For this review, take the finished solid that the model builds, in its own axes (mm). A direction names the side the tool comes from. Round coordinates to 2 decimals unless told otherwise and drop trailing zeros. Order: outer loops, then holes, each group sorted by start corner. A loop starts at its lowest first (then second) coordinate and runs counter-clockwise, first axis right, second up. Notation, with made-up numbers: (68.5, 43) -> (84.5, 43) arc R16 cw to (84.5, 70) -> close; hole circle Ø10 at (69.5, 51). An arc over 180 degrees is marked (long way). Answer in a Markdown table with one row per item.
Autodesk Inventor part; units mm, degrees
sketch "Skizze1" plane through (0, 0, 0) normal (0, 0, 1) x (1, 0, 0)
  circle A0 centre (0, 0) radius 21
  line L0 (-16.8526, 12.5296) -> (0, 0)
  line L1 (0, 0) -> (-8.33, 19.2772)
  line L2 (0, 0) -> (8.0192, 19.4086)
  line L3 (0, 0) -> (18.1865, 10.5)
  line L4 (0, 0) -> (21, 0) construction
  line L5 (0, 0) -> (-13.5496, -16.044)
  line L6 (0, 0) -> (13.0769, -16.4315)
  circle A1 centre (0, 0) radius 27.5
  circle A2 centre (0, 0) radius 12.5
  line L7 (-27.5, 11.3909) -> (-11.3909, 27.5)
  line L8 (-11.3909, 27.5) -> (11.3909, 27.5)
  line L9 (11.3909, 27.5) -> (27.5, 11.3909)
  line L10 (27.5, 11.3909) -> (27.5, -11.3909)
  line L11 (27.5, -11.3909) -> (11.3909, -27.5)
  line L12 (11.3909, -27.5) -> (-11.3909, -27.5)
  line L13 (-11.3909, -27.5) -> (-27.5, -11.3909)
  line L14 (-27.5, -11.3909) -> (-27.5, 11.3909)
  circle A3 centre (0, 0) radius 3.25
  point P0 (0, 0)
  point P1 (-27.5, 0)
  dimension "d3" = 55
  dimension "d0" = 42
  dimension "d1" = 30
  dimension "d2" = 30
  dimension "d4" = 25
  dimension "d27" = 0
  dimension "d28" = 0
  dimension "d105" = 6.5
extrude "Extrusion21" add sketch "Skizze1" along normal blind 53 contours A0 L6 A2 L3 | L3 A2 L2 A0 | A0 L5 A2 L6 | L2 A2 L1 A0 | A2 L6 A3 L3 | L3 A3 L2 A2 | A0 L0 A2 L5 | A2 L5 A3 L6 | L1 A2 L0 A0 | L2 A3 L1 A2 | A3 L6 L3 | L3 L2 A3 | A2 L0 A3 L5 | A3 L5 L6 | L1 A3 L0 A2 | L2 L1 A3 | L5 A3 L0 | L0 A3 L1 | A1 | L10 L11 A1 | A1 L9 L10 | A1 L8 L9 | L11 L12 A1 | A1 L7 L8 | L12 L13 A1 | A1 L14 L7 | L13 L14 A1
sketch "Skizze18" plane through (0, 0, 0) normal (0, 0, 1) x (1, 0, 0)
  line L0 (-11.3909, 27.5) -> (11.3909, 27.5)
  line L1 (-11.3909, 27.5) -> (63.1653, 27.5)
  line L2 (63.1653, 27.5) -> (63.1653, -27.5)
  line L3 (63.1653, -27.5) -> (-11.3909, -27.5)
  line L4 (-11.3909, -27.5) -> (-11.3909, 27.5)
  point P0 (0, 0)
  dimension "d154" = 55
extrude "Extrusion22" cut sketch "Skizze18" along normal through all
sketch "Skizze19" plane through (0, 0, 0) normal (1, 0, 0) x (0, 1, 0)
  line L0 (12.25, 9.875) -> (-12.25, 9.875)
  line L1 (-12.25, 9.875) -> (-12.25, 5.125)
  line L2 (-12.25, 5.125) -> (12.25, 5.125)
  line L3 (12.25, 5.125) -> (12.25, 9.875)
  line L4 (27.5, 0) -> (-27.5, 0)
  line L5 (-27.5, 0) -> (-27.5, 53)
  point P0 (0, 0)
  dimension "d157" = 24.5
  dimension "d158" = 4.75
  dimension "d159" = 5.125
  dimension "d160" = 39.75
sketch "Skizze20" plane through (0, 0, 0) normal (1, 0, 0) x (0, 1, 0)
  line L0 (-15, 48.125) -> (15, 48.125)
  line L1 (15, 48.125) -> (15, 42.875)
  line L2 (15, 42.875) -> (-15, 42.875)
  line L3 (-15, 42.875) -> (-15, 48.125)
  line L4 (5, 48.125) -> (-5, 48.125)
  line L5 (-5, 48.125) -> (-5, 42.875)
  line L6 (-5, 42.875) -> (5, 42.875)
  line L7 (5, 42.875) -> (5, 48.125)
  line L8 (-27.5, 53) -> (27.5, 53)
  point P0 (0, 0)
  dimension "d165" = 30
  dimension "d166" = 5.25
  dimension "d168" = 10
  dimension "d169" = 5.25
  dimension "d170" = 10
  dimension "d171" = 5
  dimension "d172" = 4.875
extrude "Extrusion23" cut sketch "Skizze20" against normal blind 20.5 contours L0 L5 L2 L3 | L0 L1 L2 L7
extrude "Extrusion25" add sketch "Skizze19" along normal blind 10 and the other way blind 25
fillet "Rundung11" radius 2 5 edges at (-19.4454, 19.4454, 53) (-27.5, 0, 53) (-19.4454, -19.4454, 53) (-27.5, -11.3909, 26.5) (-27.5, 11.3909, 26.5)
fillet "Rundung12" radius 1 12 edges at (-11.3909, 15, 45.5) (-11.3909, 10, 42.875) (-11.3909, 5, 45.5) (-11.3909, 10, 48.125) (-11.3909, -5, 45.5) (-11.3909, -10, 42.875) (-11.3909, -15, 45.5) (-11.3909, -10, 48.125) (10, 0, 9.875) (10, -12.25, 7.5) (10, 0, 5.125) (10, 12.25, 7.5)
sketch "Skizze22" plane through (0, 0, 0) normal (0, 1, 0) x (-1, 0, 0)
  line L0 (26.9142, 0) -> (11.3909, 0)
  line L1 (11.3909, 0) -> (11.3909, 51)
  line L2 (11.3909, 53) -> (25.5, 53)
  line L3 (-11.1091, 37.75) -> (-11.1091, 15.25)
  line L4 (11.3909, 15.25) -> (11.3909, 37.75)
  line L5 (11.3909, 37.75) -> (2.2757, 37.75)
  line L6 (-2.494, 37.75) -> (-11.1091, 37.75)
  arc A0 (-2.494, 37.75) -> (-2.494, 15.25) centre (-0.1091, 26.5) ccw
  arc A1 (2.2757, 15.25) -> (2.2757, 37.75) centre (-0.1091, 26.5) ccw
  line L7 (-11.1091, 15.25) -> (-2.494, 15.25)
  line L8 (2.2757, 15.25) -> (11.3909, 15.25)
  line L9 (11.3909, 0) -> (11.3909, 51)
  point P0 (0, 0)
  point P1 (11.3909, 26.5)
  dimension "d195" = 26.5
  dimension "d196" = 11.5
  dimension "d197" = 22.5
  dimension "d198" = 22.5
  dimension "d199" = 15.25
  dimension "d200" = 0
extrude "Extrusion26" cut sketch "Skizze1" along normal blind 20 contours A3 L6 L3 | L3 L2 A3 | A3 L5 L6 | L2 L1 A3 | L5 A3 L0 | L0 A3 L1
extrude "Extrusion28" add sketch "Skizze22" along normal mid plane 55 contours L8 A1 L1 | A1 L5 L1
sketch "Skizze12" plane through (0, 0, 14.5) normal (0, 0, 1) x (1, 0, 0)
  circle A0 centre (0, 0) radius 21
  line L0 (-16.8526, 12.5296) -> (-10.0313, 7.4581)
  line L1 (-4.9583, 11.4745) -> (-8.33, 19.2772)
  line L2 (4.7734, 11.5527) -> (8.0192, 19.4086)
  line L3 (10.8253, 6.25) -> (18.1865, 10.5)
  line L4 (0, 0) -> (21, 0) construction
  line L5 (-8.0652, -9.55) -> (-13.5496, -16.044)
  line L6 (7.7839, -9.7807) -> (13.0769, -16.4315)
  circle A1 centre (0, 0) radius 27.5
  circle A2 centre (0, 0) radius 12.5
  line L7 (-27.5, 11.3909) -> (-11.3909, 27.5)
  line L8 (-11.3909, 27.5) -> (11.3909, 27.5)
  line L9 (11.3909, 27.5) -> (27.5, 11.3909)
  line L10 (27.5, 11.3909) -> (27.5, -11.3909)
  line L11 (27.5, -11.3909) -> (11.3909, -27.5)
  line L12 (11.3909, -27.5) -> (-11.3909, -27.5)
  line L13 (-11.3909, -27.5) -> (-27.5, -11.3909)
  line L14 (-27.5, -11.3909) -> (-27.5, 11.3909)
  point P0 (0, 0)
  point P1 (-27.5, 0)
  dimension "d91" = 55
  dimension "d88" = 42
  dimension "d89" = 30
  dimension "d90" = 30
  dimension "d92" = 25
  dimension "d93" = 0
  dimension "d94" = 0
sketch "Skizze13" plane through (0, -27.5, 0) normal (0, 1, 0) x (-1, 0, 0)
  circle A0 centre (0, 41) radius 11.5
  line L0 (-38.5, 14.5) -> (38.5, 14.5)
  line L1 (27.5, 0) -> (27.5, 67.5)
  point P0 (0, 0)
  point P1 (27.5, 14.5)
  dimension "d100" = 23
  dimension "d101" = 26.5
  dimension "d102" = 27.5
sketch "Skizze14" plane through (0, 0, 0) normal (0, 1, 0) x (-1, 0, 0)
  line L0 (11.3909, 42.5805) -> (11.3909, 39.4195)
  line L1 (27.5, 67.5) -> (11.3909, 67.5)
  line L2 (11.3909, 67.5) -> (11.3909, 14.5)
  line L3 (11.3909, 14.5) -> (27.5, 14.5)
  line L4 (27.5, 14.5) -> (27.5, 67.5)
  arc A0 (11.3909, 42.5805) -> (-11.3909, 42.5805) centre (0, 41) ccw
  line L5 (0, 52.5) -> (11.3909, 52.5)
  line L6 (11.3909, 52.5) -> (11.3909, 29.5)
  line L7 (11.3909, 29.5) -> (0, 29.5)
  line L8 (0, 29.5) -> (0, 52.5)
  point P0 (0, 0)
  dimension "d108" = 23
  dimension "d111" = 25
  dimension "d112" = 5.25
  dimension "d113" = 5.375
  dimension "d114" = 40
  dimension "d115" = 30
  dimension "d116" = 4.75
  dimension "d117" = 4.875
  dimension "d124" = 10
  dimension "d125" = 4.75
  dimension "d126" = 10
sketch "Skizze16" plane through (-11.391, 0, 0) normal (1, 0, 0) x (0, 1, 0)
  line L0 (-12.5, 25.125) -> (12.5, 25.125)
  line L1 (12.5, 25.125) -> (12.5, 19.875)
  line L2 (12.5, 19.875) -> (-12.5, 19.875)
  line L3 (-12.5, 19.875) -> (-12.5, 25.125)
  line L4 (-15, 62.125) -> (15, 62.125)
  line L5 (15, 62.125) -> (15, 57.375)
  line L6 (15, 57.375) -> (-15, 57.375)
  line L7 (-15, 57.375) -> (-15, 62.125)
  line L8 (5, 62.125) -> (-5, 62.125)
  line L9 (-5, 62.125) -> (-5, 57.375)
  line L10 (-5, 57.375) -> (5, 57.375)
  line L11 (5, 57.375) -> (5, 62.125)
  point P0 (0, 0)
  dimension "d130" = 25
  dimension "d131" = 5.25
  dimension "d134" = 30
  dimension "d135" = 4.75
  dimension "d137" = 10
  dimension "d138" = 4.75
  dimension "d139" = 10
  dimension "d144" = 42
  dimension "d145" = 30
  dimension "d146" = 30
  dimension "d148" = 25
  dimension "d149" = 0
  dimension "d150" = 0
  dimension "d151" = 6.5
sketch "Skizze2" plane through (0, 0, 14.5) normal (0, 0, 1) x (1, 0, 0)
  circle A0 centre (0, 0) radius 21
  line L0 (-16.8526, 12.5296) -> (0, 0)
  line L1 (0, 0) -> (-8.33, 19.2772)
  line L2 (0, 0) -> (8.0192, 19.4086)
  line L3 (0, 0) -> (18.1865, 10.5)
  line L4 (0, 0) -> (21, 0) construction
  line L5 (0, 0) -> (-13.5496, -16.044)
  line L6 (0, 0) -> (13.0769, -16.4315)
  circle A1 centre (0, 0) radius 27.5
  circle A2 centre (0, 0) radius 12.5
  point P0 (0, 0)
  dimension "d11" = 42
  dimension "d12" = 30
  dimension "d13" = 30
  dimension "d14" = 55
  dimension "d15" = 25
  dimension "d29" = 0
  dimension "d30" = 0
sketch "Skizze3" plane through (0, 0, 48) normal (0, 0, 1) x (1, 0, 0)
  circle A0 centre (0, 0) radius 3.25
  dimension "d19" = 6.5
  dimension "d38" = 0
sketch "Skizze6" plane through (0, 0, 14.5) normal (0, 0, 1) x (1, 0, 0)
  circle A0 centre (0, 0) radius 21
  line L0 (-16.8526, 12.5296) -> (0, 0)
  line L1 (0, 0) -> (-8.33, 19.2772)
  line L2 (0, 0) -> (8.0192, 19.4086)
  line L3 (0, 0) -> (18.1865, 10.5)
  line L4 (0, 0) -> (21, 0) construction
  line L5 (0, 0) -> (-13.5496, -16.044)
  line L6 (0, 0) -> (13.0769, -16.4315)
  circle A1 centre (0, 0) radius 27.5
  circle A2 centre (0, 0) radius 12.5
  line L7 (5.2672, -3.0014) -> (0.0343, -6.0622)
  line L8 (0.0343, -6.0622) -> (-5.2328, -3.0608)
  line L9 (-5.2328, -3.0608) -> (-5.2672, 3.0014)
  line L10 (-5.2672, 3.0014) -> (-0.0343, 6.0622)
  line L11 (-0.0343, 6.0622) -> (5.2328, 3.0608)
  line L12 (5.2328, 3.0608) -> (5.2672, -3.0014)
  point P0 (0, 0)
  dimension "d31" = 42
  dimension "d32" = 30
  dimension "d33" = 30
  dimension "d34" = 55
  dimension "d35" = 25
  dimension "d36" = 0
  dimension "d37" = 0
  dimension "d39" = 10.5
sketch "Skizze7" plane through (0, 0, 48) normal (0, 0, 1) x (1, 0, 0)
  circle A0 centre (0, 0) radius 27.5
  line L0 (27.5, -11.3909) -> (11.3909, -27.5)
  line L1 (11.3909, -27.5) -> (-11.3909, -27.5)
  line L2 (-11.3909, -27.5) -> (-27.5, -11.3909)
  line L3 (-27.5, -11.3909) -> (-27.5, 11.3909)
  line L4 (-27.5, 11.3909) -> (-11.3909, 27.5)
  line L5 (-11.3909, 27.5) -> (11.3909, 27.5)
  line L6 (11.3909, 27.5) -> (27.5, 11.3909)
  line L7 (27.5, 11.3909) -> (27.5, -11.3909)
  point P0 (0, 0)
  point P1 (0, 0)
  point P2 (27.5, 0)
  dimension "d45" = 23
  dimension "d46" = 16.5
  dimension "d47" = 43.125
sketch "Skizze9" plane through (27.5, -11.3909, 48) normal (1, 0, 0) x (0, 0, -1)
  circle A0 centre (16.5, 27.0159) radius 9.5
  line L0 (0, 22.7817) -> (0, 0)
  line L1 (0, -16.1091) -> (48, -16.1091)
  point P0 (-48, 11.3909)
  dimension "d49" = 19
  dimension "d52" = 16.5
  dimension "d53" = 43.125
sketch "Skizze10" plane through (27.5, -11.3909, 48) normal (1, 0, 0) x (0, 0, -1)
  line L0 (25, 43.6027) -> (8, 43.6027)
  line L1 (8, 43.6027) -> (8, 26.6027)
  line L2 (8, 26.6027) -> (25, 26.6027)
  line L3 (25, 26.6027) -> (25, 43.6027)
  ellipse E0 centre (16.5, 26.6027) end of major axis (16.5, 37.9638) minor radius 11.3535 (27.1922, 22.7817) -> (5.8078, 22.7817) ccw
  point P0 (48, 11.3909)
  dimension "d58" = 17
  dimension "d59" = 17
  dimension "d60" = 17
  dimension "d61" = 8.5
equation "\"d169\" = d166"
equation "\"d196\" = 0.5 * d194"
equation "\"d125\" = d116"
equation "\"d138\" = d135"
equation "\"d52\" = d46"
equation "\"d53\" = d47"
properties part number "Stangenbereich_2"
Q1. Clearance check with flat-ended pins moving along their axes: pin 1 Ø4 at (x, z) = (-18, 44.5) entering from -Y; pin 2 Ø12 at (y, z) = (9, 45.5) entering from +X; pin 3 Ø12 at (x, y) = (-14, -0.5) entering from -Z; pin 4 Ø4 at (y, z) = (10, 46.5) entering from +X. State where each tip first meets the part, or that it passes through.
Answer key:
| item | result |
|---|---|
| pin 1 | stops at y = -22.89 |
| pin 2 | stops at x = -11.39 |
| pin 3 | stops at z = 0 |
| pin 4 | stops at x = -11.61 |
Q2. The part is to be moulded in two halves that separate along Y. For faces 6 (the face through (-20.5, 10, 46)), 7 (the face through (-19.04, -19.85, 25.14)), 8 (the face through (-9, 27.5, 18)), say which applies: +Y half, -Y half, draft (parallel to the pull), parting line (faces both ways), or undercut.
Answer key:
| item | result |
|---|---|
| face 6 | undercut |
| face 7 | -Y half |
| face 8 | +Y half |
Q3. Take a section at C-C, the plane z = 41. Write out the cut boundary in (x, y).
Answer key:
| item | result |
|---|---|
| outline | (-27.5, -10.56) arc R2 ccw to (-26.91, -11.98) -> (-11.39, -27.5) -> (-11.39, 27.5) -> (-26.91, 11.98) arc R2 ccw to (-27.5, 10.56) -> close |
Q4. Take a section at B-B, the plane x = 0. Write out the cut boundary in (y, z) (3 decimals).
Answer key:
| item | result |
|---|---|
| outline | (-12.25, 5.125) -> (-3.25, 5.125) -> (-3.25, 9.875) -> (-12.25, 9.875) -> close; (3.25, 5.125) -> (12.25, 5.125) -> (12.25, 9.875) -> (3.25, 9.875) -> close |
Q5. To check wall thickness, follow probe 1 along X at (y, z) = (0, 8.8); probe 2 along Y at (x, z) = (-14, 46); probe 3 along Y at (x, z) = (0, 7.95). State the ranges of each line that lie inside material, in increasing order.
Answer key:
| item | result |
|---|---|
| probe 1 | x = -27.5 to -3.25, 3.25 to 10 |
| probe 2 | y = -24.89 to -15, -5 to 5, 15 to 24.89 |
| probe 3 | y = -12.25 to -3.25, 3.25 to 12.25 |
Q6. Take a section at A-A, the plane y = 0. Write out the cut boundary in (x, z) (3 decimals), then the cut area to 3 significant figures.
Answer key:
| item | result |
|---|---|
| outline | (-27.5, 0) -> (-11.391, 0) -> (-11.391, 5.125) -> (-3.25, 5.125) -> (-3.25, 9.875) -> (-11.391, 9.875) -> (-11.391, 15.25) -> (-2.276, 15.25) arc R11.5 cw to (-2.276, 37.75) -> (-11.391, 37.75) -> (-11.391, 53) -> (-25.5, 53) arc R2 ccw to (-27.5, 51) -> close; (3.25, 5.125) -> (9, 5.125) arc R1 ccw to (10, 6.125) -> (10, 8.875) arc R1 ccw to (9, 9.875) -> (3.25, 9.875) -> close |
| area | 975 mm^2 |
Q7. Take a section at D-D, the plane y = -7. Write out the cut boundary in (x, z) (3 decimals), then the cut area to 3 significant figures.
Answer key:
| item | result |
|---|---|
| outline | (-27.5, 0) -> (-11.391, 0) -> (-11.391, 5.125) -> (9, 5.125) arc R1 ccw to (10, 6.125) -> (10, 8.875) arc R1 ccw to (9, 9.875) -> (-11.391, 9.875) -> (-11.391, 15.25) -> (-2.276, 15.25) arc R11.5 cw to (-2.276, 37.75) -> (-11.391, 37.75) -> (-11.391, 41.875) arc R1 ccw to (-12.391, 42.875) -> (-20.5, 42.875) -> (-20.5, 48.125) -> (-12.391, 48.125) arc R1 ccw to (-11.391, 49.125) -> (-11.391, 53) -> (-25.5, 53) arc R2 ccw to (-27.5, 51) -> close |
| area | 958 mm^2 |
Q8. Tool access review of faces 1 (the face through (-16, -10, 48.125)), 2 (the face through (-11.391, 0, 45)), 3 (the face through (-9, -27.5, 18)), 4 (the face through (-7, 0, 15.25)), 5 (the face through (-1, 12.25, 7)): name each direction out of +Z, -Z, +X, -X, +Y, -Y from which nothing blocks a thin tool from reaching the whole face with its end or side.
Answer key:
| item | result |
|---|---|
| face 1 | +X |
| face 2 | +Z, +X, +Y, -Y |
| face 3 | +Z, -Z, +X, -X, -Y |
| face 4 | +X, +Y, -Y |
| face 5 | -Z, +X, +Y |
